Solid Edge part; units mm, degrees
sketch "Sketch1" plane through (0, 0, 0) normal (0, 0, 1) x (1, 0, 0)
  line L0 (0, 15) -> (117.75, 15)
  line L1 (117.75, -15) -> (0, -15)
  arc A0 (117.75, 15) -> (117.75, -15) centre (117.75, 0) cw
  arc A1 (0, -15) -> (0, 15) centre (0, 0) cw
extrude "Protrusion1" add sketch "Sketch1" against normal blind 20
sketch "Sketch2" plane through (103.5, 0, 0) normal (0, 0, 1) x (1, 0, 0)
  circle A0 centre (-103.5, 0) radius 7.5
  circle A1 centre (14.25, 0) radius 7.5
extrude "ExtrudedProtrusion_2" add sketch "Sketch2" along normal blind 40
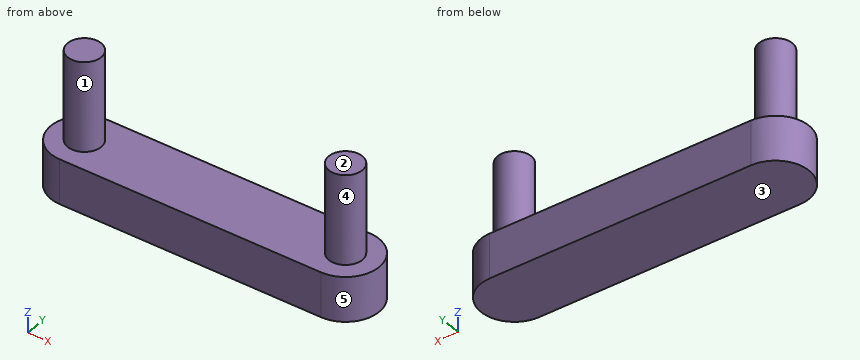
Geometry check sheet. Reference: the model listing, model coordinates, mm. Face numbers are marked on the shaded views. A direction names the side the tool comes from. Give positions to 0.01 mm unless a question says otherwise; leave off trailing zeros. Order: outer loops, then holes, each group sorted by start corner. A loop starts at its lowest first (then second) coordinate and runs counter-clockwise, first axis right, second up.
1. Access from +Z, -Z, +X, -X, +Y, -Y to the whole of each face (thin tool, end or side, straight path). Record for the marked faces 1 and 2.
2. Section check A-A, the plane y = 0. Enter the section's corners in (x, z).
3. Release check for a two-part mould opening along X. For the marked faces 3, 4 and 5 record: pulls with the +X half, pulls with the -X half, needs draft (parallel to the pull), parting line crosses it, or undercut.
4. Thickness scan on L1, parallel to Z at x = 83, y = -12.25; L2, parallel to X at y = 3.5, z = 33.5; L3, parallel to X at y = 5.75, z = 18.5. Record the ranges inside material, lowest first.
5. Section check C-C, the plane z = 20. Enter the section's corners in (x, y), and give its area (3 significant figures).
6. Gauge pin test, flat ends, axial feed: pin 1 Ø1.5 at (y, z) = (-6.5, -5.5) entering from +X; pin 2 Ø5 at (y, z) = (3, 7.5) entering from -X; pin 3 Ø10 at (x, z) = (15.5, 22) entering from +Y. Record the tip position at first contact, or that the pin passes through.
7. Section check B-B, the plane x = 44. Enter the section's corners in (y, z).
8. Section check D-D, the plane z = -9. Enter the section's corners in (x, y).
Values follow:
1. face 1: +Z
1. face 2: +Z, +X, -X, +Y, -Y
2. outline: (-15, -20) - (132.75, -20) - (132.75, 0) - (125.25, 0) - (125.25, 40) - (110.25, 40) - (110.25, 0) - (7.5, 0) - (7.5, 40) - (-7.5, 40) - (-7.5, 0) - (-15, 0) - close
3. face 3: needs draft
3. face 4: undercut
3. face 5: pulls with the +X half
4. L1: z = -20 to 0
4. L2: x = -6.63 to 6.63, 111.12 to 124.38
4. L3: x = -4.82 to 4.82, 112.93 to 122.57
5. outline: circle Ø15 at (0, 0); circle Ø15 at (117.75, 0)
5. area: 353 mm2
6. pin 1: stops at x = 131.6
6. pin 2: stops at x = -7.48
6. pin 3: passes through
7. outline: (-15, -20) - (15, -20) - (15, 0) - (-15, 0) - close
8. outline: (0, -15) - (117.75, -15) arc R15 ccw to (117.75, 15) - (0, 15) arc R15 ccw to start
